Geometry: final body of the model. Coordinates: model frame, mm. Face numbers are marked on the shaded views. A direction names the side the tool comes from. Give positions to 0.01 mm unless a question says otherwise; leave off trailing zeros. Order: outer loops, then holes, each group sorted by start corner. A loop starts at its lowest first (then second) coordinate and runs counter-clockwise, first axis right, second up. Notation, with made-up numbers: (8, 0.25) -> (43, 0.25) arc R15 ccw to (43, 18.25) -> close; hole circle Ø4 at (52.5, 17). An arc over 180 degrees is marked (long way). Answer in a Markdown table with one row per item. Add a question column.
Q1. Pull-direction query (Z, two-part tool) for the marked faces 1, 2 and 3; classes: +Z half, -Z half, draft (parallel to the pull), parting line (faces both ways), or undercut.
Q2. Contact query for flat-ended pins moving along their axis: P1, Ø1, axis at y = -0.5, z = 2, coming from the +X side; P2, Ø1.3, axis at x = -7, y = -2, coming from the -Z side; P3, Ø0.5, axis at x = -7, y = -2.5, coming from the +Z side. Output: stop coordinate, or through.
Q3. Set-up query: the marked faces 4, 5, 6, 7 and 8. Return all of +Z, -Z, +X, -X, +Y, -Y with unobstructed straight access to the full face (end or side cutting, diameter ignored); none if empty.
Q4. Cut plane A-A on z = -2.75. Return the cut outline in (x, y), and give its area (3 significant figures).
Q5. Cut plane B-B on x = 11.5. Return the cut outline in (y, z).
Q6. Line query: line 1 along Z through (x, y) = (12.5, -2.25); line 2 along Z through (x, y) = (13, -0.25); line 3 along X through (y, z) = (-2.8, -4). Output: solid intervals per line, ascending. Write a range as from..to.
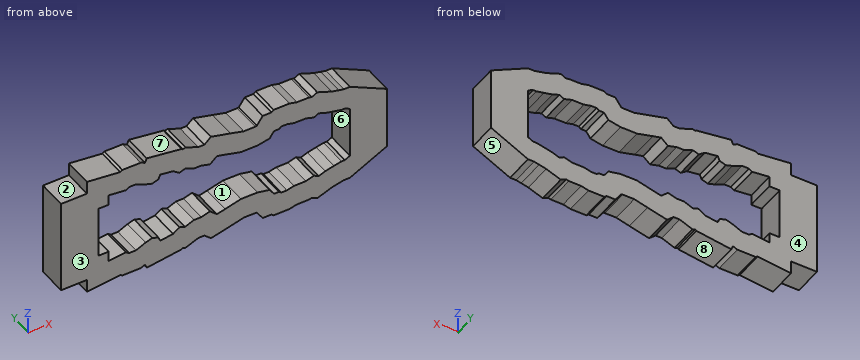
from build123d import *

# Parameters (mm, degrees)
F1_DEPTH = 4


with BuildPart() as f1:
    # F0 (on Front) → F1 (new body)
    with BuildSketch(Plane.XZ):
        Polygon((28.140141, 1.079267), (23.027079, 3.635797), (22.190165, 3.635797), (21.487397, 3.784869), (20.508261, 4.01677), (18.511227, 4.774267), (17.754608, 4.377944), (17.395179, 4.490907), (15.688958, 4.490907), (14.675495, 4.744273), (12.493739, 4.744273), (12.177031, 4.490907), (10.975377, 4.490907), (10.159982, 3.332186), (9.944286, 3.287419), (9.713922, 3.287419), (8.356896, 3.287419), (6.529206, 3.764208), (3.825945, 4.440023), (2.928981, 3.632755), (2.91847, 3.635797), (2.070995, 3.635797), (0.314703, 4.356327), (-0.052348, 4.224189), (-0.22679, 4.353405), (-5.04288, 5.041418), (-5.2829, 4.471371), (-5.886157, 4.744273), (-8.405054, 4.744273), (-8.692273, 4.549374), (-13.301984, 5.071807), (-13.301984, 3.287419), (-16.88024, 3.287419), (-16.88024, -0.282654), (-16.88024, -6.282654), (-16.88024, -9.852727), (-13.301984, -9.852727), (-13.301984, -11.637115), (-8.692273, -11.114682), (-8.405054, -11.309581), (-5.886157, -11.309581), (-5.2829, -11.036679), (-5.04288, -11.606726), (-0.22679, -10.918713), (-0.052348, -10.789497), (0.314703, -10.921635), (2.070995, -10.201105), (2.91847, -10.201105), (2.928981, -10.198063), (3.825945, -11.005331), (6.529206, -10.329516), (8.356896, -9.852727), (9.713922, -9.852727), (9.944286, -9.852727), (10.159982, -9.897494), (10.975377, -11.056215), (12.177031, -11.056215), (12.493739, -11.309581), (14.675495, -11.309581), (15.688958, -11.056215), (17.395179, -11.056215), (17.754608, -10.943252), (18.511227, -11.339575), (20.508261, -10.582078), (21.487397, -10.350178), (22.190165, -10.201105), (23.027079, -10.201105), (28.140141, -7.644575), align=None)
        Polygon((-11.733841, -6.852727), (-11.733841, 0.287419), (-10.301984, 0.287419), (-10.301984, 1.712602), (-7.926678, 1.443401), (-7.483288, 1.744273), (-6.533165, 1.744273), (-5.202995, 1.142529), (-4.284543, 0.857492), (-3.429434, 1.142529), (-3.176068, 1.744273), (-1.402506, 1.490907), (-0.547397, 0.857492), (0.244372, 1.142529), (1.479531, 0.635797), (2.492994, 0.635797), (3.696482, 0.287419), (4.646604, 1.142529), (5.786751, 0.857492), (7.972032, 0.287419), (9.713922, 0.287419), (10.252325, 0.287419), (11.930874, 0.635797), (12.532617, 1.490907), (13.229374, 1.490907), (13.546081, 1.744273), (14.306178, 1.744273), (15.319642, 1.490907), (16.934849, 1.490907), (18.043324, 1.142529), (18.708412, 1.490907), (19.626861, 1.142529), (20.83035, 0.857492), (21.875484, 0.635797), (22.318875, 0.635797), (23.015631, 0.287419), (23.015631, -6.852727), (22.318875, -7.201105), (21.875484, -7.201105), (20.83035, -7.422801), (19.626861, -7.707837), (18.708412, -8.056215), (18.043324, -7.707837), (16.934849, -8.056215), (15.319642, -8.056215), (14.306178, -8.309581), (13.546081, -8.309581), (13.229374, -8.056215), (12.532617, -8.056215), (11.930874, -7.201105), (10.252325, -6.852727), (9.713922, -6.852727), (7.972032, -6.852727), (5.786751, -7.422801), (4.646604, -7.707837), (3.696482, -6.852727), (2.492994, -7.201105), (1.479531, -7.201105), (0.244372, -7.707837), (-0.547397, -7.422801), (-1.402506, -8.056215), (-3.176068, -8.309581), (-3.429434, -7.707837), (-4.284543, -7.422801), (-5.202995, -7.707837), (-6.533165, -8.309581), (-7.483288, -8.309581), (-7.926678, -8.008709), (-10.301984, -8.27791), (-10.301984, -6.852727), align=None, mode=Mode.SUBTRACT)
    extrude(amount=F1_DEPTH)


solid = f1.part
Completed:
| question | item | result |
|---|---|---|
| 1 | face 1 | undercut |
| 1 | face 2 | +Z half |
| 1 | face 3 | draft |
| 2 | P1 | stops at x = 27.3 |
| 2 | P2 | stops at z = -11.31 |
| 2 | P3 | stops at z = 4.74 |
| 3 | face 4 | +Z, -Z, +X, -X, +Y |
| 3 | face 5 | -Z, +X, +Y, -Y |
| 3 | face 6 | +Y, -Y |
| 3 | face 7 | +Z, +Y, -Y |
| 3 | face 8 | -Z, +Y, -Y |
| 4 | outline | (-16.88, -4) -> (-11.73, -4) -> (-11.73, 0) -> (-16.88, 0) -> close; (23.02, -4) -> (28.14, -4) -> (28.14, 0) -> (23.02, 0) -> close |
| 4 | area | 41.1 mm² |
| 5 | outline | (-4, -11.06) -> (0, -11.06) -> (0, -7.11) -> (-4, -7.11) -> close; (-4, 0.55) -> (0, 0.55) -> (0, 4.49) -> (-4, 4.49) -> close |
| 6 | line 1 | z = -11.31..-8.01, 1.44..4.74 |
| 6 | line 2 | z = -11.31..-8.06, 1.49..4.74 |
| 6 | line 3 | x = -16.88..-11.73, 23.02..28.14 |
